Work out the finished part from the listing and answer in its coordinate system (mm). Coordinates: 2 decimals unless noted, no trailing zeros. Write each loop counter-clockwise with the first axis right and the second up, starting at its lowest first coordinate (ties: lowest second). Pieces come first, ordered by that corner, then holes. Notation, with made-up numbers: M 10.25,47 L 69.25,47 A13 ccw 69.25,66 Z; hole C 32,16.25 d7. An arc over 180 degrees is marked long. Answer as CSV lines item,"result". Start each with the question number.
(1) A flat-ended cylindrical pin translates along its axis: P1, Ø1, axis at y = 4.5, z = -3.5, coming from the +X side. Find the tip coordinate at first contact, or state that the pin passes through.
(2) Find the intervals of material crossed by L1, parallel to X at y = 3.95, z = -3; L2, parallel to Z at x = 0.25, y = 4.05; L3, parallel to Z at x = 1, y = 3.45, in increasing order. Write a range as [from, to].
(3) A cutting plane is placed at A-A on y = 2. Give the vertices of the cut face in (x, z).
from build123d import *

# Parameters (mm, degrees)
ESQUISSE2_OUTSIDE_W     = 25.68
ESQUISSE2_OUTSIDE_H     = 25.68
ENL_V_MAT_EXTRU_1_DEPTH = 5


with BuildPart() as part:
    # Esquisse1 → Base-Révolution (revolve)
    with BuildSketch(Plane.XY, mode=Mode.PRIVATE) as base_r_volution_sk:
        Polygon((4, 5), (6.5, 5), (9.192388155, 3.445548946), (9.192388155, 1.554451054), (6.5, 0), (4, 0), align=None)
    revolve(base_r_volution_sk.sketch.rotate(Axis((0, 2.4, 0), (0, -1, 0)), 90), axis=Axis((0, 2.4, 0), (0, -1, 0)))  # turned: the seam where the file's is

    # Esquisse2 outside → Enlèv. mat.-Extru.1 (cut)
    with BuildSketch(Plane(origin=(0, 0, 0), x_dir=(1, 0, 0), z_dir=(0, 1, 0))):
        Rectangle(ESQUISSE2_OUTSIDE_W, ESQUISSE2_OUTSIDE_H)
        Polygon((-3.75277675, -6.5), (3.75277675, -6.5), (7.505553499, 0), (3.75277675, 6.5), (-3.75277675, 6.5), (-7.505553499, 0), align=None, mode=Mode.SUBTRACT)
    extrude(amount=ENL_V_MAT_EXTRU_1_DEPTH, mode=Mode.SUBTRACT)


solid = part.part
Here are the results:
1,P1,"stops at x = 5.77"
2,L1,"x = [-5.77, -2.65], [2.65, 5.77]"
2,L2,"z = [-6.5, -3.99], [3.99, 6.5]"
2,L3,"z = [-6.5, -3.87], [3.87, 6.5]"
3,outline,"M -7.51,0 L -3.75,-6.5 L 3.75,-6.5 L 7.51,0 L 3.75,6.5 L -3.75,6.5 Z; hole C 0,0 d8"
